Answer from the drawing. Dimensions are ordinates in mm from the lowest x, y and z of the part. Round coordinates to 2 decimals unless told otherwise and drop trailing zeros. Loops run counter-clockwise (first coordinate to the right, second up) from the corner with the lowest first, then second, coordinate; pieces in that order, holes last. Notation, with made-up numbers: M 56.5,22 L 60.5,22 A21 ccw 60.5,51 Z; hole C -36.5,69.25 d6. An arc over 180 degrees is marked long. Answer as a JSON object with one key per item and string values.
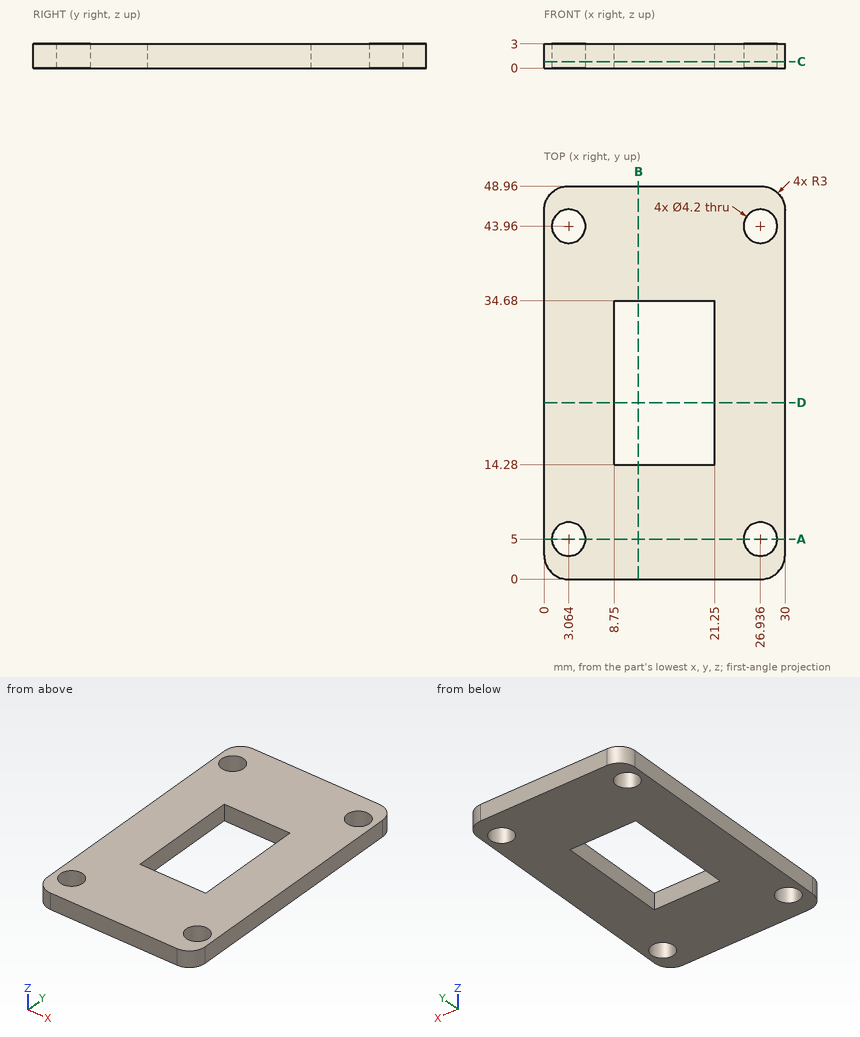
Item 1: The part is cut by section A-A (y = 5). Give the vertices of the cut face in (x, z).
Values follow:
{"outline": "M 0,0 L 0.96,0 L 0.96,3 L 0,3 Z; M 5.16,0 L 24.84,0 L 24.84,3 L 5.16,3 Z; M 29.04,0 L 30,0 L 30,3 L 29.04,3 Z"}
Item 2: The part is cut by section D-D (y = 22). Give the vertices of the cut face in (x, z).
Values follow:
{"outline": "M 0,0 L 8.75,0 L 8.75,3 L 0,3 Z; M 21.25,0 L 30,0 L 30,3 L 21.25,3 Z"}
Item 3: Straight lines are drawn through the part: line 1 (Y direction, x = 3, z = 2.8); line 2 (Y direction, x = 15.25, z = 2.5); line 3 (X direction, y = 32.5, z = 2.5). For each, find the intervals that lie inside material, in ascending order.
Values follow:
{"line 1": "0 to 2.9, 7.1 to 41.86, 46.06 to 48.96", "line 2": "0 to 14.28, 34.68 to 48.96", "line 3": "0 to 8.75, 21.25 to 30"}
Item 4: The part is cut by section C-C (z = 0.8). Give the vertices of the cut face in (x, y), then the cut area to 3 significant figures.
Values follow:
{"outline": "M 0,3 A3 ccw 3,0 L 27,0 A3 ccw 30,3 L 30,45.96 A3 ccw 27,48.96 L 3,48.96 A3 ccw 0,45.96 Z; hole C 3.06,5 d4.2; hole C 3.06,43.96 d4.2; hole M 8.75,14.28 L 21.25,14.28 L 21.25,34.68 L 8.75,34.68 Z; hole C 26.94,5 d4.2; hole C 26.94,43.96 d4.2", "area": "1,150 mm^2"}
Item 5: A flat-ended cylindrical pin translates along its axis: P1, Ø4, axis at x = 26.94, y = 43.96, coming from the +Z side. Find the tip coordinate at first contact, or state that the pin passes through.
Values follow:
{"P1": "through"}
Item 6: The part is cut by section B-B (x = 11.75). Give the vertices of the cut face in (y, z).
Values follow:
{"outline": "M 0,0 L 14.28,0 L 14.28,3 L 0,3 Z; M 34.68,0 L 48.96,0 L 48.96,3 L 34.68,3 Z"}
